For this review, take the finished solid that the model builds, in its own axes (mm). Face numbers are marked on the shaded views. Give positions to 0.01 mm unless a question says otherwise; leave off trailing zeros. Write each loop counter-clockwise with the first axis right and the second up, starting at its lowest first coordinate (ties: lowest second). Pieces come first, ordered by that corner, then holes. Notation, with made-up numbers: M -39,5.5 L 8,5.5 A16 cw 8,28.5 Z; hole C -10,66.5 d9. An arc over 180 degrees is marked long. Answer as a JSON object with one key per item and string values. Group by question number.
```python
from build123d import *

# Parameters (mm, degrees)
BOSS_EXTRUDE1_DEPTH = 4
SKETCH3_R           = 11.5
CUT_EXTRUDE1_DEPTH  = 40.855495589
SKETCH4_R           = 1.625
CUT_EXTRUDE2_DEPTH  = 40.855495589
BOSS_EXTRUDE2_DEPTH = 5.575
SKETCH7_R           = 2.1
CUT_EXTRUDE3_DEPTH  = 6
FILLET1_R           = 6


with BuildPart() as part:
    # Sketch1 → Boss-Extrude1 (new body)
    with BuildSketch(Plane(origin=(0, 0, 0), x_dir=(1, 0, 0), z_dir=(0, 1, 0))):
        Polygon((21.510162675, -33.313262079), (-20.489837325, -31.733061767), (-20.489837325, 31.733061767), (21.510162675, 33.313262079), align=None)
    extrude(amount=BOSS_EXTRUDE1_DEPTH)

    # Sketch3 → Cut-Extrude1 (cut, through all)
    with BuildSketch(Plane(origin=(0, 4, 0), x_dir=(1, 0, 0), z_dir=(0, 1, 0))):
        with Locations(Location((0, 0, 0), (0, 0, 270))):
            Circle(SKETCH3_R)
    extrude(amount=-CUT_EXTRUDE1_DEPTH, mode=Mode.SUBTRACT)

    # Sketch4 → Cut-Extrude2 (cut, through all)
    with BuildSketch(Plane(origin=(0, 4, 0), x_dir=(1, 0, 0), z_dir=(0, 1, 0))):
        with Locations(Location((-15.5, 15.5, 0), (0, 0, 270))):
            Circle(SKETCH4_R)
        with Locations(Location((15.5, 15.5, 0), (0, 0, 270))):
            Circle(SKETCH4_R)
        with Locations(Location((15.5, -15.5, 0), (0, 0, 270))):
            Circle(SKETCH4_R)
        with Locations(Location((-15.5, -15.5, 0), (0, 0, 270))):
            Circle(SKETCH4_R)
    extrude(amount=-CUT_EXTRUDE2_DEPTH, mode=Mode.SUBTRACT)

    # Sketch6 → Boss-Extrude2 (add)
    with BuildSketch(Plane.XZ.offset(-4)):
        Polygon((-20.489837325, 22), (-20.489837325, 31.733061767), (21.510162675, 33.313262079), (21.510162675, 22), align=None)
    boss_extrude2 = extrude(amount=-BOSS_EXTRUDE2_DEPTH)

    # Mirror1: Boss-Extrude2 across plane
    add(boss_extrude2.mirror(Plane.XY))

    # Sketch7 → Cut-Extrude3 (cut)
    with BuildSketch(Plane(origin=(0, 9.575, 0), x_dir=(1, 0, 0), z_dir=(0, 1, 0))):
        with Locations(Location((13.340455159, 27.331724457, 0), (0, 0, 270))):
            Circle(SKETCH7_R)
        with Locations(Location((-13.640455159, 26.316599626, 0), (0, 0, 270))):
            Circle(SKETCH7_R)
        with Locations(Location((-13.640455159, -26.316599626, 0), (0, 0, 270))):
            Circle(SKETCH7_R)
        with Locations(Location((13.340455159, -27.331724457, 0), (0, 0, 270))):
            Circle(SKETCH7_R)
    extrude(amount=-CUT_EXTRUDE3_DEPTH, mode=Mode.SUBTRACT)

    # Fillet1
    fillet1_edges = [part.edges().sort_by_distance(p)[0] for p in [
        (-20.489837325, 4.7875, -31.733061767),
        (21.510162675, 4.7875, -33.313262079),
        (21.510162675, 4.7875, 33.313262079),
        (-20.489837325, 4.7875, 31.733061767),
    ]]
    fillet(fillet1_edges, radius=FILLET1_R)


solid = part.part
```
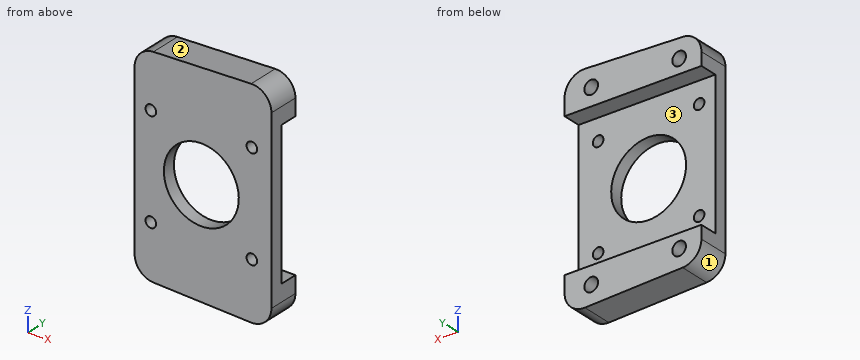
Item 1: Consider section A-A (z = 15.5). Give the boundary of the cut face in (x, y) (3 decimals), plus the area to 3 significant figures.
Item 2: Insertion check: P1, Ø5, axis at x = -15.5, z = 15.5, coming from the +Y side; P2, Ø3.5, axis at x = -13.64, z = -26.32, coming from the +Y side (3 decimals); P3, Ø14, axis at x = 0, z = 0, coming from the +Y side; P4, Ø1, axis at x = 10, y = 7, coming from the -Z side. Each pin has a flat end and moves straight along its axis. Give the tip position at first contact, or say it passes through.
Item 3: Consider section B-B (y = 7.5). Give the boundary of the cut face in (x, z).
Item 4: Consider section D-D (y = 2.25). Give the boundary of the cut face in (x, z) (3 decimals).
Item 5: Draft analysis for pull direction Z (two halves, no side actions). For the marked faces 1, 2 and 3, state which applies: released by +Z, released by -Z, zero draft, split by the parting line, or undercut.
Item 6: Consider section C-C (x = -9). Give the boundary of the cut face in (y, z) (3 decimals).
Item 7: To check wall thickness, follow probe 1 along X at (y, z) = (2.05, -15.5) (3 decimals); probe 2 along Z at (x, y) = (14, 6); probe 3 along Y at (x, z) = (-11.5, -13). State the ranges of each line that lie inside material, in increasing order.
Result set:
{
 "1": {"outline": "M -20.49,0 L -17.125,0 L -17.125,4 L -20.49,4 Z; M -13.875,0 L 13.875,0 L 13.875,4 L -13.875,4 Z; M 17.125,0 L 21.51,0 L 21.51,4 L 17.125,4 Z", "area": "142 mm^2"},
 "2": {"P1": "stops at y = 4", "P2": "stops at y = 3.575", "P3": "passes through", "P4": "stops at z = -32.9"},
 "3": {"outline": "M -20.49,-25.95 A6 ccw -14.72,-31.95 L 15.28,-33.08 A6 ccw 21.51,-27.08 L 21.51,-22 L -20.49,-22 Z; M -20.49,22 L 21.51,22 L 21.51,27.08 A6 ccw 15.28,33.08 L -14.72,31.95 A6 ccw -20.49,25.95 Z; hole C -13.64,-26.32 d4.2; hole C -13.64,26.32 d4.2; hole C 13.34,-27.33 d4.2; hole C 13.34,27.33 d4.2"},
 "4": {"outline": "M -20.49,-25.955 A6 ccw -14.715,-31.95 L 15.285,-33.079 A6 ccw 21.51,-27.083 L 21.51,27.083 A6 ccw 15.285,33.079 L -14.715,31.95 A6 ccw -20.49,25.955 Z; hole C -15.5,-15.5 d3.25; hole C -15.5,15.5 d3.25; hole C 0,0 d23; hole C 15.5,-15.5 d3.25; hole C 15.5,15.5 d3.25"},
 "5": {"face 1": "released by -Z", "face 2": "released by +Z", "face 3": "undercut"},
 "6": {"outline": "M 0,-32.165 L 9.575,-32.165 L 9.575,-22 L 4,-22 L 4,-7.159 L 0,-7.159 Z; M 0,7.159 L 4,7.159 L 4,22 L 9.575,22 L 9.575,32.165 L 0,32.165 Z"},
 "7": {"probe 1": "x = -20.49 to -17.125, -13.875 to 13.875, 17.125 to 21.51", "probe 2": "z = -33.03 to -29.33, -25.34 to -22, 22 to 25.34, 29.33 to 33.03", "probe 3": "y = 0 to 4"}
}
